The model under review builds one solid part; all positions refer to its coordinate system, in mm. Face numbers are marked on the shaded views. A direction names the side the tool comes from. Round coordinates to 2 decimals unless told otherwise and drop trailing zeros. Write each loop counter-clockwise with the first axis right and the second up, starting at its lowest first coordinate (ties: lowest second). Pieces come first, ordered by that corner, then holes. Notation, with made-up numbers: (39, 9.25) - (89, 9.25) arc R8 cw to (89, 22.25) - close; hole circle Ø11 at (82.25, 57). An arc over 180 degrees is marked (long way). Return JSON: item names as keys, results as strings.
from build123d import *

# Parameters (mm, degrees)
SKETCH1_W           = 32
SKETCH1_H           = 29
BOSS_EXTRUDE1_DEPTH = 6
SKETCH2_R           = 1
CUT_EXTRUDE1_DEPTH  = 10
SKETCH3_W           = 21
SKETCH3_H           = 9.6
CUT_EXTRUDE2_DEPTH  = 10
SKETCH4_W           = 31
SKETCH4_H           = 27
CUT_EXTRUDE3_DEPTH  = 1
FILLET2_R           = 3
SKETCH5_R           = 2
CUT_EXTRUDE4_DEPTH  = 2
CHAMFER2_SIZE       = 1
SKETCH6_W           = 1
SKETCH6_H           = 11
CUT_EXTRUDE5_DEPTH  = 2.5
FILLET3_R           = 0.3
SKETCH7_W           = 31
SKETCH7_H           = 13
CUT_EXTRUDE6_DEPTH  = 2.5
FILLET4_R           = 1
SKETCH_1_W          = 21
SKETCH_1_H          = 12.05
CUT_EXTRUDE_1_DEPTH = 2.5
FILLET_1_R          = 1
SKETCH_2_W          = 11
SKETCH_2_H          = 2.5
CUT_EXTRUDE_2_DEPTH = 33.802439001
FILLET_2_R          = 0.3


with BuildPart() as part:
    # Sketch1 → Boss-Extrude1 (new body)
    with BuildSketch(Plane(origin=(0, 0, 0), x_dir=(1, 0, 0), z_dir=(0, 1, 0))):
        Rectangle(SKETCH1_W, SKETCH1_H)
    extrude(amount=BOSS_EXTRUDE1_DEPTH)

    # Sketch2 → Cut-Extrude1 (cut)
    with BuildSketch(Plane(origin=(0, 6, 0), x_dir=(1, 0, 0), z_dir=(0, 1, 0))):
        with Locations(Location((-13, 9, 0), (0, 0, 270))):
            Circle(SKETCH2_R)
        with Locations(Location((13, 9, 0), (0, 0, 270))):
            Circle(SKETCH2_R)
        with Locations(Location((13, -9, 0), (0, 0, 270))):
            Circle(SKETCH2_R)
        with Locations(Location((-13, -9, 0), (0, 0, 270))):
            Circle(SKETCH2_R)
    extrude(amount=-CUT_EXTRUDE1_DEPTH, mode=Mode.SUBTRACT)

    # Sketch3 → Cut-Extrude2 (cut)
    with BuildSketch(Plane(origin=(0, 6, 0), x_dir=(1, 0, 0), z_dir=(0, 1, 0))):
        with Locations((0, 6.25)):
            Rectangle(SKETCH3_W, SKETCH3_H)
        with Locations((0, -6.25)):
            Rectangle(SKETCH3_W, SKETCH3_H)
    extrude(amount=-CUT_EXTRUDE2_DEPTH, mode=Mode.SUBTRACT)

    # Sketch4 → Cut-Extrude3 (cut)
    with BuildSketch(Plane.XZ):
        Rectangle(SKETCH4_W, SKETCH4_H)
    extrude(amount=-CUT_EXTRUDE3_DEPTH, mode=Mode.SUBTRACT)

    # Fillet2
    # the kernel refuses this fillet: 3 mm, written as the material it takes off along each edge
    with BuildSketch(Plane(origin=(16, 6, 22), x_dir=(0, -1, 0), z_dir=(0, 0, -1)), Plane(origin=(-16, 6, -22), x_dir=(0, -1, 0), z_dir=(0, 0, 1))) as fillet2_piece_1:
        with BuildLine():
            CenterArc((FILLET2_R, FILLET2_R), FILLET2_R, 180, 90)
            Line((0, FILLET2_R), (0, 0))
            Line((0, 0), (FILLET2_R, 0))
        make_face()
    extrude(amount=44, mode=Mode.SUBTRACT)

    # Sketch5 → Cut-Extrude4 (cut)
    with BuildSketch(Plane(origin=(0, 6, 0), x_dir=(1, 0, 0), z_dir=(0, 1, 0))):
        with Locations(Location((-13, 9, 0), (0, 0, 270))):
            Circle(SKETCH5_R)
        with Locations(Location((13, 9, 0), (0, 0, 270))):
            Circle(SKETCH5_R)
        with Locations(Location((13, -9, 0), (0, 0, 270))):
            Circle(SKETCH5_R)
        with Locations(Location((-13, -9, 0), (0, 0, 270))):
            Circle(SKETCH5_R)
    extrude(amount=-CUT_EXTRUDE4_DEPTH, mode=Mode.SUBTRACT)

    # Chamfer2
    chamfer2_edges = [part.edges().sort_by_distance(p)[0] for p in [
        (-16, 1.5, 14.5),
        (-16, 1.5, -14.5),
        (0, 6, -14.5),
        (16, 1.5, -14.5),
        (15.121320344, 5.121320344, -14.5),
        (-15.121320344, 5.121320344, -14.5),
        (0, 6, 14.5),
        (16, 1.5, 14.5),
        (15.121320344, 5.121320344, 14.5),
        (-15.121320344, 5.121320344, 14.5),
    ]]
    chamfer(chamfer2_edges, length=CHAMFER2_SIZE)

    # Sketch6 → Cut-Extrude5 (cut)
    with BuildSketch(Plane.XZ):
        with Locations((-15.5, 0)):
            Rectangle(SKETCH6_W, SKETCH6_H)
        with Locations((15.5, 0)):
            Rectangle(SKETCH6_W, SKETCH6_H)
    extrude(amount=-CUT_EXTRUDE5_DEPTH, mode=Mode.SUBTRACT)

    # Fillet3
    fillet3_edges = [part.edges().sort_by_distance(p)[0] for p in [
        (-15.5, 2.5, 5.5),
        (-15.5, 2.5, -5.5),
        (15.5, 2.5, -5.5),
        (15.5, 2.5, 5.5),
    ]]
    fillet(fillet3_edges, radius=FILLET3_R)

    # Sketch7 → Cut-Extrude6 (cut)
    with BuildSketch(Plane.XZ.offset(-1)):
        Rectangle(SKETCH7_W, SKETCH7_H)
    extrude(amount=-CUT_EXTRUDE6_DEPTH, mode=Mode.SUBTRACT)

    # Fillet4
    fillet4_edges = [part.edges().sort_by_distance(p)[0] for p in [
        (-13, 3.5, 6.5),
        (13, 3.5, 6.5),
        (-13, 3.5, -6.5),
        (13, 3.5, -6.5),
    ]]
    fillet(fillet4_edges, radius=FILLET4_R)

    # Эскиз1 → Вырез-Вытянуть1 (cut)
    with BuildSketch(Plane.XZ.offset(-1)):
        with Locations((0, -7.475)):
            Rectangle(SKETCH_1_W, SKETCH_1_H)
    extrude(amount=-CUT_EXTRUDE_1_DEPTH, mode=Mode.SUBTRACT)

    # Скругление1
    fillet_1_edges = [part.edges().sort_by_distance(p)[0] for p in [
        (10.5, 3.5, -12.275),
        (-10.5, 3.5, -12.275),
    ]]
    fillet(fillet_1_edges, radius=FILLET_1_R)

    # Эскиз2 → Вырез-Вытянуть2 (cut, through all)
    with BuildSketch(Plane.XY.offset(-13.5)):
        with Locations((0, 1.25)):
            Rectangle(SKETCH_2_W, SKETCH_2_H)
    extrude(amount=-CUT_EXTRUDE_2_DEPTH, mode=Mode.SUBTRACT)

    # Скругление2
    fillet_2_edges = [part.edges().sort_by_distance(p)[0] for p in [
        (5.5, 2.5, -14),
        (-5.5, 2.5, -14),
    ]]
    fillet(fillet_2_edges, radius=FILLET_2_R)


solid = part.part
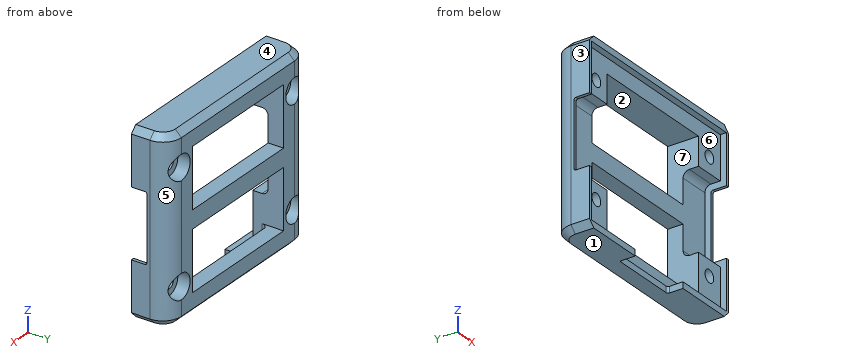
(1) Wall thickness on line 1 (X direction, y = 2.95, z = 9); line 2 (Z direction, x = -3.5, y = 4); line 3 (X direction, y = 0.75, z = -8): over which ranges is each line inside the solid? List them lowest first.
Filled in:
{"line 1": "x = -16 to -14, -12 to -10.5, 10.5 to 12, 14 to 16", "line 2": "z = -14.5 to -11.05, -1.45 to 1.45, 11.05 to 14.5", "line 3": "x = -16 to -15.5, 15.5 to 16"}
(2) Add section A-A (z = 4.25). Write out the cut boundary in (x, y), plus the area to 3 significant figures.
Filled in:
{"outline": "(-16, 2.5) - (-15.5, 2.5) - (-15.5, 3.5) - (-10.5, 3.5) - (-10.5, 6) - (-13, 6) arc R3 ccw to (-16, 3) - close; (10.5, 3.5) - (15.5, 3.5) - (15.5, 2.5) - (16, 2.5) - (16, 3) arc R3 ccw to (13, 6) - (10.5, 6) - close", "area": "24.6 mm2"}
(3) Add section C-C (z = -9). Write out the cut boundary in (x, y).
Filled in:
{"outline": "(-16, 0) - (-15.5, 0) - (-15.5, 1) - (-14, 1) - (-14, 4) - (-15, 4) - (-15, 5.24) arc R3 ccw to (-16, 3) - close; (-12, 1) - (-10.5, 1) - (-10.5, 6) - (-11, 6) - (-11, 4) - (-12, 4) - close; (10.5, 1) - (12, 1) - (12, 4) - (11, 4) - (11, 6) - (10.5, 6) - close; (14, 1) - (15.5, 1) - (15.5, 0) - (16, 0) - (16, 3) arc R3 ccw to (15, 5.24) - (15, 4) - (14, 4) - close"}
(4) For the marked faces 5, 6 and 7, list the 3-axis set-ups (+Z, -Z, +X, -X, +Y, -Y) from which the entire face can be reached by the end or side of a thin tool; tool diameter is ignored.
Filled in:
{"face 5": "+Z, -Z, +X, +Y", "face 6": "-Y", "face 7": "+Y, -Y"}
(5) Mouldability with a two-part tool opening along Z and no side actions: class the marked faces 1, 2, 3 and 4 as released by +Z, released by -Z, zero draft, split by the parting line, or undercut.
Filled in:
{"face 1": "released by -Z", "face 2": "undercut", "face 3": "zero draft", "face 4": "released by +Z"}
(6) Clearance check with flat-ended pins moving along their axes: pin 1 Ø9 at (x, z) = (3, -1.5) entering from -Y; pin 2 Ø5 at (x, z) = (2.5, 4) entering from -Y; pin 3 Ø3 at (x, z) = (13, 9) entering from -Y; pin 4 Ø0.5 at (x, y) = (4, 0.5) entering from -Z. State where each tip first meets the part, or that it passes through.
Filled in:
{"pin 1": "stops at y = 3.5", "pin 2": "passes through", "pin 3": "stops at y = 1", "pin 4": "stops at z = 13.5"}
(7) Add section D-D (x = 7). Write out the cut boundary in (y, z), plus the area to 3 significant figures.
Filled in:
{"outline": "(0, -14.5) - (5, -14.5) - (6, -13.5) - (6, -11.05) - (3.5, -11.05) - (3.5, -13.5) - (0, -13.5) - close; (0, 13.5) - (1, 13.5) - (1, 11.05) - (6, 11.05) - (6, 13.5) - (5, 14.5) - (0, 14.5) - close; (3.5, -1.45) - (6, -1.45) - (6, 1.45) - (3.5, 1.45) - close", "area": "36.6 mm2"}
(8) Add section B-B (x = 3). Write out the cut boundary in (y, z).
Filled in:
{"outline": "(0, 13.5) - (1, 13.5) - (1, 11.05) - (6, 11.05) - (6, 13.5) - (5, 14.5) - (0, 14.5) - close; (2.5, -14.5) - (5, -14.5) - (6, -13.5) - (6, -11.05) - (3.5, -11.05) - (3.5, -13.5) - (2.5, -13.5) - close; (3.5, -1.45) - (6, -1.45) - (6, 1.45) - (3.5, 1.45) - close"}
